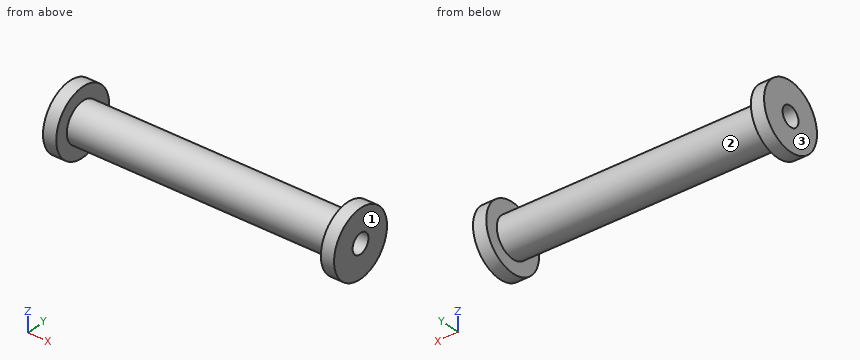
from build123d import *

# Parameters (mm, degrees)
F0_R     = 3
F1_DEPTH = 40
F2_R     = 5
F2_R_2   = 3
F3_DEPTH = 2
F4_R     = 5
F4_R_2   = 3
F5_DEPTH = 2
F6_R     = 1.5
F7_DEPTH = 44


with BuildPart() as f1:
    # F0 (on Right) → F1 (new body)
    with BuildSketch(Plane.YZ):
        with Locations((-6.2035736628, 2.2626414429)):
            Circle(F0_R)
    extrude(amount=F1_DEPTH)

    # F2 (on face) → F3 (join)
    with BuildSketch(Plane.YZ.offset(40)):
        with Locations((-6.2035736628, 2.2626414429)):
            Circle(F2_R)
        with Locations((-6.2035736628, 2.2626414429)):
            Circle(F2_R_2, mode=Mode.SUBTRACT)
        with Locations((-6.2035736628, 2.2626414429)):
            Circle(F2_R_2)
    extrude(amount=F3_DEPTH)

    # F4 (on face) → F5 (join)
    with BuildSketch(Plane(origin=(0, 0, 0), x_dir=(0, -1, 0), z_dir=(-1, 0, 0))):
        with Locations((6.2035736628, 2.2626414429)):
            Circle(F4_R)
        with Locations((6.2035736628, 2.2626414429)):
            Circle(F4_R_2, mode=Mode.SUBTRACT)
        with Locations((6.2035736628, 2.2626414429)):
            Circle(F4_R_2)
    extrude(amount=F5_DEPTH)

    # F6 (on face) → F7 (cut)
    with BuildSketch(Plane.YZ.offset(42)):
        with Locations((-6.2035736628, 2.2626414429)):
            Circle(F6_R)
    extrude(amount=-F7_DEPTH, mode=Mode.SUBTRACT)


solid = f1.part
Check sheet for the modelled part. Datum: model origin and axes. Units: mm. Face numbers are marked on the shaded views. Give positions to 0.01 mm unless a question says otherwise; leave off trailing zeros. Loops run counter-clockwise (first coordinate to the right, second up) from the corner with the lowest first, then second, coordinate; pieces in that order, holes last. Notation, with made-up numbers: M -29,50.5 L 20,50.5 A30 cw 20,86.5 Z; hole C 31,54.5 d10. An arc over 180 degrees is marked long. Answer as a JSON object with one key per item and string values. Group by question number.
Q1. Go/stop test with flat-tipped pins: P1, Ø1.8, axis at y = -6.2, z = 2.26, coming from the -X side; P2, Ø3, axis at x = 37.5, y = -5.5, coming from the +Z side; P3, Ø3, axis at x = 18.5, y = -6.5, coming from the -Z side; P4, Ø4, axis at x = 4.5, z = 2, coming from the +Y side. Record where each tip stops, or that it passes through.
Q2. Cross-section at B-B on z = -2. Record the cut outline in (x, y).
Q3. Release check for a two-part mould opening along X. For the marked faces 1, 2 and 3 record: released by +X, released by -X, zero draft, split by the parting line, or undercut.
Q4. Cross-section at C-C on z = 6.5. Record the cut outline in (x, y).
Q5. Material ranges on line 1 along X through (y, z) = (-8.25, 6.5); line 2 along Z through (x, y) = (17.5, -6.25); line 3 along Z through (x, y) = (17, -6.75), recorded low to high. Write a range as [from, to].
Q6. Cross-section at D-D on y = -8.5. Record the cut outline in (x, z), then the cut area to 3 significant figures.
Q7. Cross-section at A-A on y = -5.75. Record the cut outline in (x, z).
Evaluation:
{
 "1": {"P1": "passes through", "P2": "stops at z = 5.26", "P3": "stops at z = -0.74", "P4": "stops at y = -3.2"},
 "2": {"outline": "M -2,-8.82 L 0,-8.82 L 0,-3.59 L -2,-3.59 Z; M 40,-8.82 L 42,-8.82 L 42,-3.59 L 40,-3.59 Z"},
 "3": {"face 1": "released by +X", "face 2": "undercut", "face 3": "released by -X"},
 "4": {"outline": "M -2,-8.86 L 0,-8.86 L 0,-3.55 L -2,-3.55 Z; M 40,-8.86 L 42,-8.86 L 42,-3.55 L 40,-3.55 Z"},
 "5": {"line 1": "x = [-2, 0], [40, 42]", "line 2": "z = [-0.74, 0.76], [3.76, 5.26]", "line 3": "z = [-0.69, 0.87], [3.66, 5.21]"},
 "6": {"outline": "M -2,-2.18 L 0,-2.18 L 0,0.33 L 40,0.33 L 40,-2.18 L 42,-2.18 L 42,6.7 L 40,6.7 L 40,4.19 L 0,4.19 L 0,6.7 L -2,6.7 Z", "area": "190 mm2"},
 "7": {"outline": "M -2,-2.72 L 0,-2.72 L 0,-0.7 L 40,-0.7 L 40,-2.72 L 42,-2.72 L 42,0.83 L -2,0.83 Z; M -2,3.69 L 42,3.69 L 42,7.24 L 40,7.24 L 40,5.23 L 0,5.23 L 0,7.24 L -2,7.24 Z"}
}
